Design review of the part shown in the three views and the two pictorial views. Dimensions are in mm from the part's minimum x, y and z. Round coordinates to 2 decimals unless told otherwise and drop trailing zeros. Loops run counter-clockwise (first coordinate to the right, second up) from the corner with the lowest first, then second, coordinate; pieces in that order, holes last. Notation, with made-up numbers: (24.25, 50.5) -> (49.25, 50.5) arc R11 ccw to (49.25, 61.5) -> close; hole circle Ø10 at (39, 46.5). An arc over 180 degrees is marked (long way). Write each question's results on one line, items separated by ' | '. Start each with the question number.
Item 1: For L1, parallel to Z at x = 60, y = 10; L2, parallel to Z at x = 20, y = 6.5; L3, parallel to X at y = 10.25, z = 15, list the stretches that pass through material, from the lowest coordinate up. Write a range as from..to.
Item 2: We need section C-C (y = 1). Give the boundary of the cut face in (x, z), and give its area (3 significant figures).
Item 3: We need section D-D (x = 43). Give the boundary of the cut face in (y, z), and give its area (3 significant figures).
Item 4: We need section B-B (z = 45). Give the boundary of the cut face in (x, y), and give its area (3 significant figures).
Item 5: Mouldability with a two-part tool opening along Z and no side actions: class the marked faces 1, 2 and 3 as pulls with the +Z half, pulls with the -Z half, needs draft (parallel to the pull), parting line crosses it, or undercut.
Item 6: We need section A-A (x = 20). Give the boundary of the cut face in (y, z).
Item 7: Clearance check with a flat-ended pin moving along its axis: pin 1 Ø10.5 at (x, z) = (20, 30) entering from +Y. State where the tip first meets the part, or that it passes through.
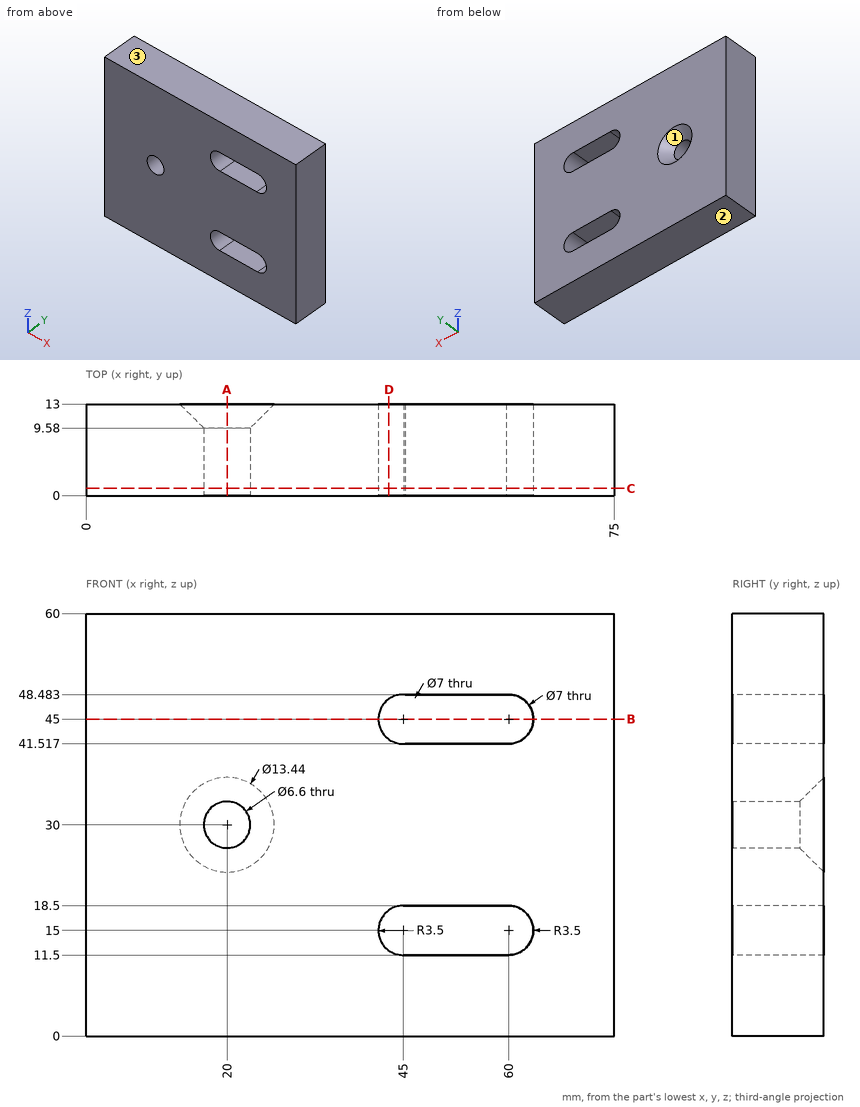
Here are the results:
1) L1: z = 0..11.5, 18.5..41.5, 48.5..60 | L2: z = 0..26.7, 33.3..60 | L3: x = 0..41.5, 63.5..75
2) outline: (0, 0) -> (75, 0) -> (75, 60) -> (0, 60) -> close; hole circle Ø6.6 at (20, 30); hole (45, 18.5) arc R3.5 ccw (long way) to (45.11, 11.5) -> (60, 11.5) arc R3.5 ccw to (60, 18.5) -> close; hole (45.34, 41.52) -> (59.66, 41.52) arc R3.5 ccw (long way) to (59.66, 48.48) -> (45.34, 48.48) arc R3.5 ccw (long way) to start | area: 4,180 mm2
3) outline: (0, 0) -> (13, 0) -> (13, 12.13) -> (0, 12.13) -> close; (0, 17.87) -> (13, 17.87) -> (13, 42.13) -> (0, 42.13) -> close; (0, 47.87) -> (13, 47.87) -> (13, 60) -> (0, 60) -> close | area: 631 mm2
4) outline: (0, 0) -> (41.5, 0) -> (41.5, 13) -> (0, 13) -> close; (63.5, 0) -> (75, 0) -> (75, 13) -> (63.5, 13) -> close | area: 689 mm2
5) face 1: undercut | face 2: pulls with the -Z half | face 3: pulls with the +Z half
6) outline: (0, 0) -> (13, 0) -> (13, 23.28) -> (9.58, 26.7) -> (0, 26.7) -> close; (0, 33.3) -> (9.58, 33.3) -> (13, 36.72) -> (13, 60) -> (0, 60) -> close
7) pin 1: stops at y = 11.53
